Geometry: final body of the model. Coordinates: model frame, mm. Face numbers are marked on the shaded views. Coordinates: 2 decimals unless noted, no trailing zeros. Write each loop counter-clockwise with the first axis right and the second up, starting at its lowest first coordinate (ties: lowest second). Pieces come first, ordered by that corner, then holes. Notation, with made-up numbers: (31.5, -2.75) - (75.5, -2.75) arc R6 ccw to (75.5, 4.25) - close; hole circle Ø6 at (32, 76). An arc over 180 degrees is marked (long way). Answer as a JSON object with one key per item and string values. Group by question number.
Item 1: Section A-A on z = 0. Return loops of the section in (x, y).
Item 2: Section C-C on y = 2.7. State how many separate pieces and enclosed holes the cut face has, and give its area (3 significant figures).
Item 3: Line query: line 1 along Z through (x, y) = (-50, 3.05); line 2 along X through (y, z) = (1.3, 0). Output: solid intervals per line, ascending. Write a range as from..to.
Item 4: Section B-B on x = -14.5. Return loops of the section in (y, z).
Item 5: Mould query, pull axis X, two halves, no side actions, for the marked faces 1 and 2. Classes: pulls with the +X half, pulls with the -X half, needs draft (parallel to the pull), parting line crosses it, or undercut.
Item 6: Section D-D on x = 9.5. Return loops of the section in (y, z).
Item 7: First-contact query: pin 1 Ø5.5 at (x, z) = (-29, 0) entering from -Y. Flat tip, straight axial feed; report the tip coordinate or a pass-through.
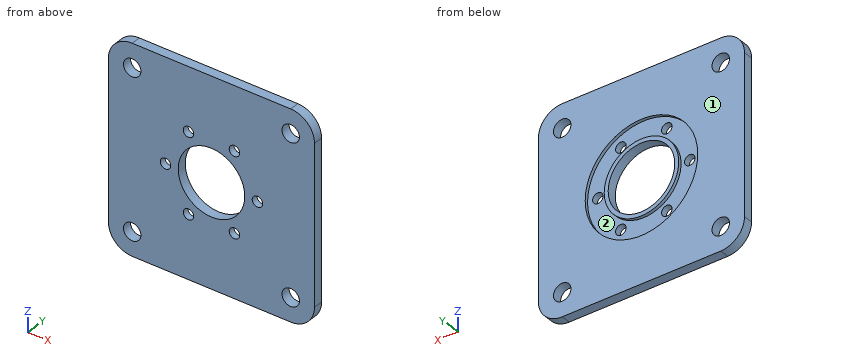
```python
from build123d import *

# Parameters (mm, degrees)
SKETCH1_R                = 21
BOSS_EXTRUDE1_DEPTH      = 6
SKETCH2_R                = 35.5
SKETCH2_R_2              = 23.5
CUT_EXTRUDE1_DEPTH       = 2
SKETCH3_R                = 5.5
CUT_EXTRUDE2_DEPTH       = 1
CUT_EXTRUDE2_DEPTH_BACK  = 7
M6_CLEARANCE_HOLE1_D     = 6.6
M6_CLEARANCE_HOLE1_DEPTH = 4
CIRPATTERN1_COUNT        = 6


with BuildPart() as part:
    # Sketch1 → Boss-Extrude1 (new body)
    with BuildSketch(Plane(origin=(0, 0, 0), x_dir=(1, 0, 0), z_dir=(0, 1, 0))):
        with BuildLine():
            Line((-50, -65), (50, -65))
            ThreePointArc((50, -65), (60.606601718, -60.606601718), (65, -50))
            Line((65, -50), (65, 50))
            ThreePointArc((65, 50), (60.606601718, 60.606601718), (50, 65))
            Line((50, 65), (-50, 65))
            ThreePointArc((-50, 65), (-60.606601718, 60.606601718), (-65, 50))
            Line((-65, 50), (-65, -50))
            ThreePointArc((-65, -50), (-60.606601718, -60.606601718), (-50, -65))
        make_face()
        Circle(SKETCH1_R, mode=Mode.SUBTRACT)
    extrude(amount=BOSS_EXTRUDE1_DEPTH)

    # Sketch2 → Cut-Extrude1 (cut)
    with BuildSketch(Plane(origin=(0, 6, 0), x_dir=(1, 0, 0), z_dir=(0, 1, 0))):
        Circle(SKETCH2_R)
        Circle(SKETCH2_R_2, mode=Mode.SUBTRACT)
    extrude(amount=-CUT_EXTRUDE1_DEPTH, mode=Mode.SUBTRACT)

    # Sketch3 → Cut-Extrude2 (cut, two sides)
    with BuildSketch(Plane(origin=(0, 6, 0), x_dir=(1, 0, 0), z_dir=(0, 1, 0))) as cut_extrude2_sk:
        with Locations((-50, 50)):
            Circle(SKETCH3_R)
        with Locations((50, 50)):
            Circle(SKETCH3_R)
        with Locations((50, -50)):
            Circle(SKETCH3_R)
        with Locations((-50, -50)):
            Circle(SKETCH3_R)
    extrude(amount=CUT_EXTRUDE2_DEPTH, mode=Mode.SUBTRACT)
    extrude(cut_extrude2_sk.sketch, amount=-CUT_EXTRUDE2_DEPTH_BACK, mode=Mode.SUBTRACT)

    # M6 Clearance Hole1
    with Locations(Plane(origin=(-29, 4, 0), x_dir=(0, 0, 1), z_dir=(0, 1, 0))):
        with Locations((0, 0)):
            m6_clearance_hole1 = Hole(M6_CLEARANCE_HOLE1_D / 2, depth=M6_CLEARANCE_HOLE1_DEPTH)

    # CirPattern1: M6 Clearance Hole1 ×6 about axis
    cirpattern1_axis = Axis((0, 0, 0), (0, 1, 0))
    for i in range(1, CIRPATTERN1_COUNT):
        add(m6_clearance_hole1.rotate(cirpattern1_axis, i * 360 / CIRPATTERN1_COUNT), mode=Mode.SUBTRACT)


solid = part.part
```
Checks:
{
 "1": {"outline": "(-65, 0) - (-32.3, 0) - (-32.3, 4) - (-35.5, 4) - (-35.5, 6) - (-65, 6) - close; (-25.7, 0) - (-21, 0) - (-21, 6) - (-23.5, 6) - (-23.5, 4) - (-25.7, 4) - close; (21, 0) - (25.7, 0) - (25.7, 4) - (23.5, 4) - (23.5, 6) - (21, 6) - close; (32.3, 0) - (65, 0) - (65, 6) - (35.5, 6) - (35.5, 4) - (32.3, 4) - close"},
 "2": {"separate pieces": "1", "enclosed holes": "11", "area": "14,700 mm^2"},
 "3": {"line 1": "-65..-55.5, -44.5..44.5, 55.5..65", "line 2": "-65..-32.3, -25.7..-21, 21..25.7, 32.3..65"},
 "4": {"outline": "(0, -65) - (6, -65) - (6, -32.4) - (4, -32.4) - (4, -28.41) - (0, -28.41) - close; (0, -21.81) - (4, -21.81) - (4, -18.49) - (6, -18.49) - (6, -15.19) - (0, -15.19) - close; (0, 15.19) - (6, 15.19) - (6, 18.49) - (4, 18.49) - (4, 21.81) - (0, 21.81) - close; (0, 28.41) - (4, 28.41) - (4, 32.4) - (6, 32.4) - (6, 65) - (0, 65) - close"},
 "5": {"face 1": "needs draft", "face 2": "undercut"},
 "6": {"outline": "(0, -65) - (6, -65) - (6, -34.21) - (4, -34.21) - (4, -21.49) - (6, -21.49) - (6, -18.73) - (0, -18.73) - close; (0, 18.73) - (6, 18.73) - (6, 21.49) - (4, 21.49) - (4, 34.21) - (6, 34.21) - (6, 65) - (0, 65) - close"},
 "7": {"pin 1": "through"}
}
